from build123d import *

# Parameters (mm, degrees)
BOSS_EXTRUDE1_DEPTH            = 5
FILLET2_R                      = 5
M5_CLEARANCE_HOLE1_D           = 5.5
M5_CLEARANCE_HOLE1_CSINK_D     = 5.55
M5_CLEARANCE_HOLE1_CSINK_ANGLE = 90
M5_CLEARANCE_HOLE2_D           = 5.5
M5_CLEARANCE_HOLE2_CSINK_D     = 5.55
M5_CLEARANCE_HOLE2_CSINK_ANGLE = 90
M5_CLEARANCE_HOLE3_D           = 5.5
M5_CLEARANCE_HOLE3_CSINK_D     = 5.55
M5_CLEARANCE_HOLE3_CSINK_ANGLE = 90


with BuildPart() as part:
    # Sketch2 → Boss-Extrude1 (new body)
    with BuildSketch(Plane(origin=(0, 0, 0), x_dir=(1, 0, 0), z_dir=(0, 1, 0))):
        Polygon((-57.5, 0), (57.5, 0), (57.5, 20), (37.5, 20), (37.5, 40), (-37.5, 40), (-37.5, 20), (-57.5, 20), align=None)
    extrude(amount=BOSS_EXTRUDE1_DEPTH)

    # Fillet2
    fillet2_edges = [part.edges().sort_by_distance(p)[0] for p in [
        (37.5, 2.5, -20),
        (57.5, 2.5, -20),
        (57.5, 2.5, 0),
        (-57.5, 2.5, 0),
        (-57.5, 2.5, -20),
        (-37.5, 2.5, -20),
        (-37.5, 2.5, -40),
        (37.5, 2.5, -40),
    ]]
    fillet(fillet2_edges, radius=FILLET2_R)

    # M5 Clearance Hole1 (through all)
    with Locations(Plane(origin=(-27.5, 5, -30), x_dir=(0, 0, 1), z_dir=(0, 1, 0))):
        with Locations((0, 0)):
            m5_clearance_hole1 = CounterSinkHole(M5_CLEARANCE_HOLE1_D / 2, M5_CLEARANCE_HOLE1_CSINK_D / 2, counter_sink_angle=M5_CLEARANCE_HOLE1_CSINK_ANGLE)

    # Mirror1: M5 Clearance Hole1 across plane
    add(m5_clearance_hole1.mirror(Plane(origin=(0, 0, 0), x_dir=(0, 0, 1), z_dir=(1, 0, 0))), mode=Mode.SUBTRACT)

    # M5 Clearance Hole2 (through all)
    with Locations(Plane(origin=(-47.5, 5, -10), x_dir=(0, 0, 1), z_dir=(0, 1, 0))):
        with Locations((0, 0)):
            m5_clearance_hole2 = CounterSinkHole(M5_CLEARANCE_HOLE2_D / 2, M5_CLEARANCE_HOLE2_CSINK_D / 2, counter_sink_angle=M5_CLEARANCE_HOLE2_CSINK_ANGLE)

    # Mirror2: M5 Clearance Hole2 across plane
    add(m5_clearance_hole2.mirror(Plane(origin=(0, 0, 0), x_dir=(0, 0, 1), z_dir=(1, 0, 0))), mode=Mode.SUBTRACT)

    # M5 Clearance Hole3 (through all)
    with Locations(Plane(origin=(0, 5, -10), x_dir=(0, 0, 1), z_dir=(0, 1, 0))):
        with Locations((0, 0)):
            CounterSinkHole(M5_CLEARANCE_HOLE3_D / 2, M5_CLEARANCE_HOLE3_CSINK_D / 2, counter_sink_angle=M5_CLEARANCE_HOLE3_CSINK_ANGLE)


solid = part.part
Design review of the part built by this model. Coordinates are the model's own, in mm. A direction names the side the tool comes from. Round coordinates to 2 decimals unless told otherwise and drop trailing zeros. Write each loop counter-clockwise with the first axis right and the second up, starting at its lowest first coordinate (ties: lowest second). Pieces come first, ordered by that corner, then holes. Notation, with made-up numbers: (4.5, 86) - (30.5, 86) arc R18 cw to (30.5, 93) - close; hole circle Ø11 at (12, -29). An arc over 180 degrees is marked (long way). Use a Markdown table: item, result. Add a question column.
1. Clearance check with flat-ended pins moving along their axes: pin 1 (7 mm diameter, centred on x = 27.5, z = -30, fed in from +Y); pin 2 (3.5 mm diameter, centred on x = -27.5, z = -30, fed in from -Y); pin 3 (1.5 mm diameter, centred on x = -41, y = 3, fed in from -Z); pin 4 (1 mm diameter, centred on y = 2.5, z = -26.5, fed in from +X). State where each tip first meets the part, or that it passes through.
2. We need section D-D (x = -27.5). State the section outline as (y, z) points (3 decimals), then the cut area to 3 significant figures.
3. We need section A-A (x = 47.5). State the section outline as (y, z) points (3 decimals).
4. We need section B-B (z = -10). State the section outline as (x, y) points (3 decimals).
5. For faces 5 (the face through (-1, 0, -16)), 6 (the face through (-47, 2, -20)), 7 (the face through (48, 2, -20)), list the 3-axis set-ups (+Z, -Z, +X, -X, +Y, -Y) from which the entire face can be reached by the end or side of a thin tool; tool diameter is ignored.
6. Mouldability with a two-part tool opening along X and no side actions: class faces 1 (the face through (-56, 2.54, -18.57)), 2 (the face through (56.07, 2.54, -18.5)), 3 (the face through (44.773, 2.453, -9.642)), 4 (the face through (-1, 5, -16)) as +X half, -X half, draft (parallel to the pull), parting line (faces both ways), or undercut.
7. We need section C-C (y = 2.65). State the section outline as (x, z) points.
8. Wall thickness on probe 1 along X at (y, z) = (3.45, -30); probe 2 along X at (y, z) = (2.7, -10); probe 3 along Z at (x, y) = (-47.5, 1.3): over which ranges is each line inside the solid? List them lowest first.
Output:
| question | item | result |
|---|---|---|
| 1 | pin 1 | stops at y = 5 |
| 1 | pin 2 | passes through |
| 1 | pin 3 | stops at z = -20.53 |
| 1 | pin 4 | stops at x = 37.5 |
| 2 | outline | (0, -40) - (5, -40) - (5, -32.775) - (4.975, -32.75) - (0, -32.75) - close; (0, -27.25) - (4.975, -27.25) - (5, -27.225) - (5, 0) - (0, 0) - close |
| 2 | area | 172 mm2 |
| 3 | outline | (0, -20) - (5, -20) - (5, -12.775) - (4.975, -12.75) - (0, -12.75) - close; (0, -7.25) - (4.975, -7.25) - (5, -7.225) - (5, 0) - (0, 0) - close |
| 4 | outline | (-57.5, 0) - (-50.25, 0) - (-50.25, 4.975) - (-50.275, 5) - (-57.5, 5) - close; (-44.75, 0) - (-2.75, 0) - (-2.75, 4.975) - (-2.775, 5) - (-44.725, 5) - (-44.75, 4.975) - close; (2.75, 0) - (44.75, 0) - (44.75, 4.975) - (44.725, 5) - (2.775, 5) - (2.75, 4.975) - close; (50.25, 0) - (57.5, 0) - (57.5, 5) - (50.275, 5) - (50.25, 4.975) - close |
| 5 | face 5 | +Z, -Z, +X, -X, -Y |
| 5 | face 6 | -Z, -X, +Y, -Y |
| 5 | face 7 | -Z, +X, +Y, -Y |
| 6 | face 1 | -X half |
| 6 | face 2 | +X half |
| 6 | face 3 | undercut |
| 6 | face 4 | draft |
| 7 | outline | (-57.5, -15) arc R5 ccw to (-52.5, -20) - (-42.5, -20) arc R5 cw to (-37.5, -25) - (-37.5, -35) arc R5 ccw to (-32.5, -40) - (32.5, -40) arc R5 ccw to (37.5, -35) - (37.5, -25) arc R5 cw to (42.5, -20) - (52.5, -20) arc R5 ccw to (57.5, -15) - (57.5, -5) arc R5 ccw to (52.5, 0) - (-52.5, 0) arc R5 ccw to (-57.5, -5) - close; hole circle Ø5.5 at (-47.5, -10); hole circle Ø5.5 at (-27.5, -30); hole circle Ø5.5 at (0, -10); hole circle Ø5.5 at (27.5, -30); hole circle Ø5.5 at (47.5, -10) |
| 8 | probe 1 | x = -37.5 to -30.25, -24.75 to 24.75, 30.25 to 37.5 |
| 8 | probe 2 | x = -57.5 to -50.25, -44.75 to -2.75, 2.75 to 44.75, 50.25 to 57.5 |
| 8 | probe 3 | z = -20 to -12.75, -7.25 to 0 |
